Model file for the job. Use its own axes, mm. A direction names the side the tool comes from. Round coordinates to 2 decimals unless told otherwise and drop trailing zeros. Loops run counter-clockwise (first coordinate to the right, second up) from the corner with the lowest first, then second, coordinate; pieces in that order, holes last. Notation, with made-up numbers: M 43.25,58.25 L 54.25,58.25 A18 ccw 54.25,89.25 Z; hole C -25,73 d11. An arc over 180 degrees is marked long. Answer in a Markdown table with one row per item.
from build123d import *

# Parameters (mm, degrees)
SKETCH1_W                      = 100
SKETCH1_H                      = 100
BOSS_EXTRUDE1_DEPTH            = 10
BOSS_EXTRUDE2_REACH            = 214.132
BOSS_EXTRUDE2_END_MAJOR_RADIUS = 50
BOSS_EXTRUDE2_END_MINOR_RADIUS = 35
SKETCH4_R                      = 12.5
BOSS_EXTRUDE21_DEPTH           = 10
FILLET1_R                      = 1
CUT_EXTRUDE1_REACH             = 230.031
FILLET11_R                     = 1


with BuildPart() as part:
    # Sketch1 → Boss-Extrude1 (new body)
    with BuildSketch(Plane(origin=(0, 0, 0), x_dir=(1, 0, 0), z_dir=(0, 1, 0))):
        Rectangle(SKETCH1_W, SKETCH1_H)
    extrude(amount=BOSS_EXTRUDE1_DEPTH)



with BuildPart() as body_2:
    # Sweep1: sweep along a path in Sketch2
    with BuildLine(Plane(origin=(0, 210, 0), x_dir=(1, 0, 0), z_dir=(0, 1, 0))) as sweep1_path:
        ThreePointArc((0, -50), (-14.644660941, -14.644660941), (-50, 0))
    # Sketch3 → Sweep1 (sweep)
    with BuildSketch(Plane.XY.offset(50)):
        with BuildLine():
            Line((25, 210), (35, 210))
            ThreePointArc((35, 210), (0, 175), (-35, 210))
            Line((-35, 210), (-25, 210))
            ThreePointArc((-25, 210), (0, 185), (25, 210))
        make_face()
    sweep(path=sweep1_path.line)


with BuildPart() as part_1:
    add(part.part)

    add(body_2.part)  # Boss-Extrude2 merges body 2
    # Boss-Extrude2: up to this torus (the profile starts outside it)
    boss_extrude2_end = Plane(origin=(-50, 210, 50), z_dir=(0, 1, 0)) * Torus(BOSS_EXTRUDE2_END_MAJOR_RADIUS, BOSS_EXTRUDE2_END_MINOR_RADIUS, mode=Mode.PRIVATE)
    # Sketch4 → Boss-Extrude2 (add, up to the surface)
    with BuildSketch(Plane(origin=(0, 10, 0), x_dir=(1, 0, 0), z_dir=(0, 1, 0)), mode=Mode.PRIVATE) as boss_extrude2_sk1:
        with Locations(Location((-14.644660941, -14.644660941, 0), (0, 0, 134.571678601))):
            Circle(SKETCH4_R)
    boss_extrude2_tool1 = extrude(boss_extrude2_sk1.sketch, amount=BOSS_EXTRUDE2_REACH, mode=Mode.PRIVATE) - boss_extrude2_end
    add(boss_extrude2_tool1.solids().sort_by_distance((-14.644661, 10, 14.644661))[0])

    # Sketch21 → Boss-Extrude21 (add)
    with BuildSketch(Plane(origin=(14.233580657, 10, 36.500543766), x_dir=(1, 0, 0), z_dir=(0, 1, 0))):
        Polygon((-21.733580657, -13.499456234), (-31.733580657, -28.499456234), (3.266419343, -28.499456234), (-6.733580657, -13.499456234), align=None)
    extrude(amount=-BOSS_EXTRUDE21_DEPTH)

    # Fillet1
    fillet1_edges = [part_1.edges().sort_by_distance(p)[0] for p in [
        (-17.5, 5, 65),
        (17.5, 5, 65),
    ]]
    fillet(fillet1_edges, radius=FILLET1_R)

    # Sketch22 → Cut-Extrude1 (cut, up to next)
    with BuildSketch(Plane(origin=(-40.028558931, 10, 2.604903453), x_dir=(1, 0, 0), z_dir=(0, 1, 0)), mode=Mode.PRIVATE) as cut_extrude1_sk1:
        Polygon((-9.971441069, -4.895096547), (5.028558931, -14.895096547), (5.028558931, 20.104903453), (-9.971441069, 10.104903453), align=None)
    cut_extrude1_tool1 = extrude(cut_extrude1_sk1.sketch, amount=-CUT_EXTRUDE1_REACH, mode=Mode.PRIVATE) & part_1.part
    add(cut_extrude1_tool1.solids().sort_by_distance((-41.5, 10, 0))[0], mode=Mode.SUBTRACT)

    # Fillet11
    fillet11_edges = [part_1.edges().sort_by_distance(p)[0] for p in [
        (-35, 5, -17.5),
        (-35, 5, 17.5),
    ]]
    fillet(fillet11_edges, radius=FILLET11_R)


solid = part_1.part
1. Saw through at B-B (x = 44.5). Write the cut outline in (y, z).
Verdict:
| item | result |
|---|---|
| outline | M 0,-50 L 10,-50 L 10,50 L 0,50 Z |
2. Tool access for faces 4 (the flat face through (12.045, 5.07, 56.817)), 5 (the flat face through (-43.183, 5.07, -12.045)), 6 (the flat face through (-29, 5, 50)), 7 (the flat face through (-50, 5, -28)), 8 (the cylindrical face through (-22.332, 92.484, 24.502)): list every direction of +Z, -Z, +X, -X, +Y, -Y with a clear straight run to the whole face (end or side of a thin tool).
Verdict:
| item | result |
|---|---|
| face 4 | +X, +Y, -Y |
| face 5 | -Y |
| face 6 | -X, +Y, -Y |
| face 7 | +Z, -Z, -X, +Y, -Y |
| face 8 | none |
3. Mould opens along Z. For faces 1 (the flat face through (28, 5, 50)), 2 (the flat face through (-50, 184, 0)), 3 (the flat face through (-8, 185, 50)) say: +Z half, -Z half, draft (parallel to the pull), parting line (faces both ways), or undercut.
Verdict:
| item | result |
|---|---|
| face 1 | undercut |
| face 2 | draft |
| face 3 | +Z half |
4. Pin check, flat tips, straight feed: pin 1 (11 mm diameter, centred on x = 32.5, y = 7.5, fed in from +Z); pin 2 (8 mm diameter, centred on y = 161.5, z = 11.5, fed in from -X); pin 3 (12 mm diameter, centred on x = -19, y = 96, fed in from -Z). Stop position of each tip, or through.
Verdict:
| item | result |
|---|---|
| pin 1 | stops at z = 50 |
| pin 2 | stops at x = -27.14 |
| pin 3 | stops at z = 2.14 |
5. Wall check: probe 1 along Y at (x, z) = (35, 25.5); probe 2 along Y at (x, z) = (-24.5, -18); probe 3 along Y at (x, z) = (-32, -14.5). Give the ranges that are in metal, low to high.
Verdict:
| item | result |
|---|---|
| probe 1 | y = 0 to 10 |
| probe 2 | y = 0 to 10, 183.3 to 199.36 |
| probe 3 | y = 0 to 10, 179.39 to 191.64 |
6. Saw through at A-A (z = -42.5). Write the cut outline in (x, y), and give its area (3 significant figures).
Verdict:
| item | result |
|---|---|
| outline | M -50,0 L 50,0 L 50,10 L -50,10 Z |
| area | 1,000 mm² |
7. Saw through at C-C (y = 96.5). Write the cut outline in (x, z), and give its area (3 significant figures).
Verdict:
| item | result |
|---|---|
| outline | C -14.64,14.64 d25 |
| area | 491 mm² |
